```python
from build123d import *

# Parameters (mm, degrees)
BOSS_EXTRU_1_START                             = -3
ESQUISSE1_W                                    = 44
ESQUISSE1_H                                    = 64
ESQUISSE1_W_2                                  = 20.5
ESQUISSE1_H_2                                  = 40.5
BOSS_EXTRU_1_DEPTH                             = 4
BOSS_EXTRU_2_DEPTH                             = 44
ENL_V_MAT_EXTRU_1_REACH                        = 103.741
ESQUISSE3_R                                    = 8.2
ESQUISSE4_R                                    = 10.6
ESQUISSE4_R_2                                  = 8.2
BOSS_EXTRU_3_DEPTH                             = 3
CONG_1_R                                       = 4
CONG_2_R                                       = 3
ENL_V_MAT_EXTRU_2_REACH                        = 100.261
ESQUISSE5_R                                    = 2.5
ENL_V_START                                    = -2
ESQUISSE6_R                                    = 10.25
ENL_V_MAT_EXTRU_3_DEPTH                        = 2
ENL_V_MAT_EXTRU_4_REACH                        = 121.659
ESQUISSE7_R                                    = 4.95
FRAISAGE_POUR_VIS_T_TE_FRAIS_E_M31_D           = 3.4
FRAISAGE_POUR_VIS_T_TE_FRAIS_E_M31_CSINK_D     = 6.3
FRAISAGE_POUR_VIS_T_TE_FRAIS_E_M31_CSINK_ANGLE = 90


with BuildPart() as part:
    # Esquisse1 → Boss.-Extru.1 (new body)
    with BuildSketch(Plane.XY.offset(BOSS_EXTRU_1_START)):
        with Locations((-10, 0)):
            Rectangle(ESQUISSE1_W, ESQUISSE1_H)
        with Locations((-10, 0)):
            Rectangle(ESQUISSE1_W_2, ESQUISSE1_H_2, mode=Mode.SUBTRACT)
    extrude(amount=-BOSS_EXTRU_1_DEPTH)

    # Esquisse2 → Boss.-Extru.2 (add)
    with BuildSketch(Plane(origin=(12, 0, 0), x_dir=(0, 0, -1), z_dir=(1, 0, 0))):
        Polygon((3, -37.5), (92, -37.5), (92, 32), (88, 32), (88, -32), (7, -32), (7, -28.443383769), (3, -28.443383769), (3, -32), align=None)
    extrude(amount=-BOSS_EXTRU_2_DEPTH)

    # Esquisse3 → Enlèv. mat.-Extru.1 (cut, up to next)
    with BuildSketch(Plane(origin=(0, 0, -92), x_dir=(-1, 0, 0), z_dir=(0, 0, -1)), mode=Mode.PRIVATE) as enl_v_mat_extru_1_sk1:
        with Locations((10, 10)):
            Circle(ESQUISSE3_R)
    enl_v_mat_extru_1_tool1 = extrude(enl_v_mat_extru_1_sk1.sketch, amount=-ENL_V_MAT_EXTRU_1_REACH, mode=Mode.PRIVATE) & part.part
    add(enl_v_mat_extru_1_tool1.solids().sort_by_distance((-10, 10, -92))[0], mode=Mode.SUBTRACT)

    # Esquisse4 → Boss.-Extru.3 (add)
    with BuildSketch(Plane.XY.offset(-88)):
        with Locations((-10, 10)):
            Circle(ESQUISSE4_R)
        with Locations(Location((-10, 10, 0), (0, 0, 180))):
            Circle(ESQUISSE4_R_2, mode=Mode.SUBTRACT)
    extrude(amount=BOSS_EXTRU_3_DEPTH)

    # Congé1
    # the kernel refuses this fillet: 4 mm, written as the material it adds along each edge
    with BuildSketch(Plane(origin=(-10, 10, -88), x_dir=(1, 0, 0), z_dir=(0, -1, 0))) as cong_1_piece_1:
        with BuildLine():
            CenterArc((14.472983346, 4), CONG_1_R, 194.477512186, 75.522487814)
            Line((10.6, 3), (10.522540333, 2.98))
            ThreePointArc((10.522540333, 2.98), (10.52, 1.5), (10.52, 0))
            Line((10.52, 0), (10.6, -0.08))
            Line((10.6, -0.08), (14.472983346, -0.08))
            Line((14.472983346, -0.08), (14.472983346, 0))
        make_face()
    revolve(axis=Axis((-10, 10, -88), (0, 0, 1)))

    # Congé2
    cong_2_edges = [part.edges().sort_by_distance(p)[0] for p in [
        (12, 32, -90),
        (-32, 32, -90),
        (-10, -32, -88),
        (-10, -37.5, -3),
        (-10, -37.5, -92),
        (-10, -32, -7),
        (-32, 32, -5),
        (12, 32, -5),
    ]]
    fillet(cong_2_edges, radius=CONG_2_R)

    # Esquisse5 → Enlèv. mat.-Extru.2 (cut, up to next)
    with BuildSketch(Plane(origin=(0, 0, -7), x_dir=(-1, 0, 0), z_dir=(0, 0, -1)), mode=Mode.PRIVATE) as enl_v_mat_extru_2_sk1:
        with Locations((4.6, 25.8)):
            Circle(ESQUISSE5_R)
    enl_v_mat_extru_2_tool1 = extrude(enl_v_mat_extru_2_sk1.sketch, amount=-ENL_V_MAT_EXTRU_2_REACH, mode=Mode.PRIVATE) & part.part
    # Esquisse5 → Enlèv. mat.-Extru.2 (cut, up to next)
    with BuildSketch(Plane(origin=(0, 0, -7), x_dir=(-1, 0, 0), z_dir=(0, 0, -1)), mode=Mode.PRIVATE) as enl_v_mat_extru_2_sk2:
        with Locations((15.4, 25.8)):
            Circle(ESQUISSE5_R)
    enl_v_mat_extru_2_tool2 = extrude(enl_v_mat_extru_2_sk2.sketch, amount=-ENL_V_MAT_EXTRU_2_REACH, mode=Mode.PRIVATE) & part.part
    # Esquisse5 → Enlèv. mat.-Extru.2 (cut, up to next)
    with BuildSketch(Plane(origin=(0, 0, -7), x_dir=(-1, 0, 0), z_dir=(0, 0, -1)), mode=Mode.PRIVATE) as enl_v_mat_extru_2_sk3:
        with Locations((4.6, -25.8)):
            Circle(ESQUISSE5_R)
    enl_v_mat_extru_2_tool3 = extrude(enl_v_mat_extru_2_sk3.sketch, amount=-ENL_V_MAT_EXTRU_2_REACH, mode=Mode.PRIVATE) & part.part
    # Esquisse5 → Enlèv. mat.-Extru.2 (cut, up to next)
    with BuildSketch(Plane(origin=(0, 0, -7), x_dir=(-1, 0, 0), z_dir=(0, 0, -1)), mode=Mode.PRIVATE) as enl_v_mat_extru_2_sk4:
        with Locations((15.4, -25.8)):
            Circle(ESQUISSE5_R)
    enl_v_mat_extru_2_tool4 = extrude(enl_v_mat_extru_2_sk4.sketch, amount=-ENL_V_MAT_EXTRU_2_REACH, mode=Mode.PRIVATE) & part.part
    add(enl_v_mat_extru_2_tool1.solids().sort_by_distance((-4.6, 25.8, -7))[0], mode=Mode.SUBTRACT)
    add(enl_v_mat_extru_2_tool2.solids().sort_by_distance((-15.4, 25.8, -7))[0], mode=Mode.SUBTRACT)
    add(enl_v_mat_extru_2_tool3.solids().sort_by_distance((-4.6, -25.8, -7))[0], mode=Mode.SUBTRACT)
    add(enl_v_mat_extru_2_tool4.solids().sort_by_distance((-15.4, -25.8, -7))[0], mode=Mode.SUBTRACT)

    # Esquisse6 → Enlèv. mat.-Extru.3 (cut)
    with BuildSketch(Plane(origin=(0, -32, 0), x_dir=(1, 0, 0), z_dir=(0, 1, 0)).offset(ENL_V_START)):
        with Locations(Location((-10, 51, 0), (0, 0, 270))):
            Circle(ESQUISSE6_R)
    extrude(amount=ENL_V_MAT_EXTRU_3_DEPTH, mode=Mode.SUBTRACT)

    # Esquisse7 → Enlèv. mat.-Extru.4 (cut, up to next)
    with BuildSketch(Plane.XZ.offset(37.5), mode=Mode.PRIVATE) as enl_v_mat_extru_4_sk1:
        with Locations(Location((-10, -51, 0), (0, 0, 270))):
            Circle(ESQUISSE7_R)
    enl_v_mat_extru_4_tool1 = extrude(enl_v_mat_extru_4_sk1.sketch, amount=-ENL_V_MAT_EXTRU_4_REACH, mode=Mode.PRIVATE) & part.part
    add(enl_v_mat_extru_4_tool1.solids().sort_by_distance((-10, -37.5, -51))[0], mode=Mode.SUBTRACT)

    # Fraisage pour vis à tête fraisée M31 (through all)
    with Locations(Plane(origin=(0, -37.5, 0), x_dir=(-1, 0, 0), z_dir=(0, -1, 0))):
        with Locations((10, 58.5), (17.5, 51), (10, 43.5), (2.5, 51)):
            CounterSinkHole(FRAISAGE_POUR_VIS_T_TE_FRAIS_E_M31_D / 2, FRAISAGE_POUR_VIS_T_TE_FRAIS_E_M31_CSINK_D / 2, counter_sink_angle=FRAISAGE_POUR_VIS_T_TE_FRAIS_E_M31_CSINK_ANGLE)


solid = part.part
```
Geometry check sheet. Reference: the model listing, model coordinates, mm. A direction names the side the tool comes from. Coordinates: 2 decimals unless noted, no trailing zeros. Write each loop counter-clockwise with the first axis right and the second up, starting at its lowest first coordinate (ties: lowest second). Pieces come first, ordered by that corner, then holes. Notation, with made-up numbers: M 23.5,61.25 L 69.5,61.25 A30 ccw 69.5,85.25 Z; hole C 34.25,53 d10. An arc over 180 degrees is marked long. One line per item, written item: value. Start each with the question number.
(1) Release check for a two-part mould opening along Z. For faces 1 (the face through (11.1, 31.14, -89.97)), 2 (the face through (-10, -5, -88)), 3 (the face through (-10.31, -36.6, -91.14)) record: released by +Z, released by -Z, zero draft, split by the parting line, or undercut.
(2) Tool access check on faces 4 (the face through (-25, 2, -7)), 5 (the face through (-17.71, -26.76, -5.03)), 6 (the face through (-6.921, -33.014, -41.223)). Record the directions out of +Z, -Z, +X, -X, +Y, -Y that give a thin tool (end or side, any length) a straight path to the whole face; none if there is none.
(3) Depth check by flat-ended pin: pin 1 (4.5 mm diameter, centred on x = -8, z = -5.5, fed in from -Y); pin 2 (4.5 mm diameter, centred on x = -4.6, y = -25.8, fed in from +Z); pin 3 (5.5 mm diameter, centred on x = -10, z = -43.5, fed in from -Y); pin 4 (1 mm diameter, centred on x = 1.5, z = -80, fed in from +Y). Enter the tip coordinate at first touch or a pass-through.
(4) Sectioned sample at D-D, the plane y = -25.8. Enter the section's corners in (x, z).
(5) Scan lines: line 1 along Z through (x, y) = (-10, -34.65); line 2 along Z through (x, y) = (-25.5, 2.5); line 3 along Y through (x, z) = (-4, -4). Record each from-to range of solid material in increasing order. Write a range as [from, to].
(6) Sectioned sample at C-C, the plane x = 7. Enter the section's corners in (y, z), and give its area (3 significant figures).
(7) Sectioned sample at B-B, the plane z = -51. Enter the section's corners in (x, y).
(8) Sectioned sample at A-A, the plane y = 10. Enter the section's corners in (x, z).
Filled sheet:
1. face 1: zero draft
1. face 2: undercut
1. face 3: released by -Z
2. face 4: +X, -X, +Y
2. face 5: +Z
2. face 6: +Y
3. pin 1: y = -37.5
3. pin 2: z = -88
3. pin 3: y = -37.1
3. pin 4: y = -32
4. outline: M -32,-92 L 12,-92 L 12,-88 L -32,-88 Z; M -32,-7 L -17.9,-7 L -17.9,-3 L -32,-3 Z; M -12.9,-7 L -7.1,-7 L -7.1,-3 L -12.9,-3 Z; M -2.1,-7 L 12,-7 L 12,-3 L -2.1,-3 Z
5. line 1: [-92, -60.2], [-56.8, -55.95], [-46.05, -45.2], [-41.8, -3]
5. line 2: [-92, -88], [-7, -3]
5. line 3: [-36.74, -28.23], [-23.37, -20.25], [20.25, 23.37], [28.23, 32]
6. outline: M -37.5,-89 A3 ccw -34.5,-92 L 32,-92 L 32,-88 L -29,-88 A3 cw -32,-85 L -32,-10 A3 cw -29,-7 L 32,-7 L 32,-3 L -34.5,-3 A3 ccw -37.5,-6 Z
6. area: 1,000 mm²
7. outline: M -32,-37.5 L -20.65,-37.5 L -19.2,-36.05 L -19.2,-34 L -20.25,-34 L -20.25,-32 L -32,-32 Z; M -15.8,-36.05 L -14.95,-36.9 L -14.95,-34 L -15.8,-34 Z; M -5.05,-36.9 L -4.2,-36.05 L -4.2,-34 L -5.05,-34 Z; M -0.8,-36.05 L 0.65,-37.5 L 12,-37.5 L 12,-32 L 0.25,-32 L 0.25,-34 L -0.8,-34 Z
8. outline: M -32,-92 L -18.2,-92 L -18.2,-85 L -20.6,-85 A4 cw -24.47,-88 L -32,-88 Z; M -32,-7 L -20.25,-7 L -20.25,-3 L -32,-3 Z; M -1.8,-92 L 12,-92 L 12,-88 L 4.47,-88 A4 cw 0.6,-85 L -1.8,-85 Z; M 0.25,-7 L 12,-7 L 12,-3 L 0.25,-3 Z
